from build123d import *

# Parameters (mm, degrees)
F0_W      = 69.0672509372
F0_H      = 104.8798933625
F1_DEPTH  = 25.4
F2_W      = 61.0817540437
F2_H      = 44.6812286973
F3_DEPTH  = 5.08
F5_R      = 6.6887407384
F6_DEPTH  = 25.4
F7_R      = 3.582784906
F8_DEPTH  = 25.4
F9_W      = 4.2634103447
F9_H      = 5.4003186524
F9_W_2    = 5.400320515
F9_H_2    = 4.2634103447
F9_W_3    = 5.1160920411
F9_H_3    = 5.4003195837
F10_DEPTH = 2.286
F4_R      = 4.3385405976
F4_R_2    = 4.6616734777
F11_DEPTH = 2.032
F14_DEPTH = 0.635


with BuildPart() as f1:
    # F0 (on Top) → F1 (new body)
    with BuildSketch(Plane.XY):
        with Locations((-0.2842266113, 5.2582062781)):
            Rectangle(F0_W, F0_H)
    extrude(amount=F1_DEPTH)

    # F2 (on face) → F3 (cut)
    with BuildSketch(Plane.XY.offset(25.4)):
        with Locations((-0.3880532458, 30.3628817201)):
            Rectangle(F2_W, F2_H)
    extrude(amount=-F3_DEPTH, mode=Mode.SUBTRACT)

    # F5 (on Top) → F6 (join)
    with BuildSketch(Plane.XY):
        with Locations((-34.5117151737, 57.5216077268)):
            Circle(F5_R)
    extrude(amount=F6_DEPTH)

    # F7 (on face) → F8 (cut)
    with BuildSketch(Plane.XY.offset(25.4)):
        with Locations((-34.5117151737, 57.5216077268)):
            Circle(F7_R)
    extrude(amount=-F8_DEPTH, mode=Mode.SUBTRACT)

    # F9 (on face) → F10 (join)
    with BuildSketch(Plane.XY.offset(25.4)):
        with Locations((-18.1905506179, -23.1645293534)):
            Rectangle(F9_W, F9_H)
        with Locations((-23.0224160478, -18.3326648548)):
            Rectangle(F9_W_2, F9_H_2)
        with Locations((-18.1905506179, -18.3326648548)):
            Rectangle(F9_W, F9_H_2)
        with Locations((-13.5007994249, -18.3326648548)):
            Rectangle(F9_W_3, F9_H_2)
        with Locations((-18.1905506179, -13.5007998906)):
            Rectangle(F9_W, F9_H_3)
    extrude(amount=F10_DEPTH)

    # F4 (on face) → F11 (join)
    with BuildSketch(Plane.XY.offset(25.4)):
        with Locations((7.2477986105, -11.08486671)):
            Circle(F4_R)
        with Locations((18.3326639235, -4.2634103447)):
            Circle(F4_R_2)
    extrude(amount=F11_DEPTH)

    # F12 (on face) + F13 (on face) → F14 (join)
    with BuildSketch(Plane.XY.offset(25.4)):
        Polygon((5.6323851459, -22.5031040609), (4.3169683777, -21.1328770965), (-1.1299567856, -25.4363407869), (0, -26.8878247589), align=None)
    with BuildSketch(Plane.XY.offset(25.4)):
        Polygon((-10.0978044793, -26.4493525028), (-4.3428572826, -21.790586412), (-5.4735084007, -20.5657135335), (-11.1444314917, -25.1564601203), align=None)
    extrude(amount=F14_DEPTH)


solid = f1.part
The listing builds one solid part. Answer for the finished solid, in the listing's coordinates (mm). A direction names the side the tool comes from. Give positions to 0.01 mm unless a question says otherwise; leave off trailing zeros. Loops run counter-clockwise (first coordinate to the right, second up) from the corner with the lowest first, then second, coordinate; pieces in that order, holes last. Notation, with made-up numbers: (3, -7) - (36, -7) arc R33 ccw to (36, 28) - close; hole circle Ø6 at (-22, 63). An arc over 180 degrees is marked (long way). Use one line per item in the form item = value.
1. Which of the six approach directions +Z, -Z, +X, -X, +Y, -Y give full straight-line access (tool end or side, diameter ignored) to faces 5 (the face through (-18, -10.801, 27)), 6 (the face through (0, 52.703, 23)), 7 (the face through (-39.038, 62.446, 12.522)), 8 (the face through (-13, -16.201, 27)), 9 (the face through (2, -24, 26.035))?
Calculated:
face_5 = +Z, -X, +Y
face_6 = +Z
face_7 = +Z, -Z
face_8 = +Z, +X, +Y
face_9 = +Z, +X, -Y
2. Find the intervals of material crossed by line 1 along Y through (x, z) = (11, 23.75); line 2 along Y through (x, z) = (-4, 11.75); line 3 along Z through (x, y) = (-14, 26), in increasing order. Write a range as [from, to].
Calculated:
line_1 = [-47.18, 8.02], [52.7, 57.7]
line_2 = [-47.18, 57.7]
line_3 = [0, 20.32]
3. Given pin 1 Ø6 at (x, z) = (-16.5, 4) entering from +Y; pin 2 Ø1.8 at (y, z) = (-19.5, 27) entering from -X; pin 3 Ø0.7 at (y, z) = (-13, 27) entering from -X, each flat-ended and moving along its own axis, determine where each tip first touches the part or whether it passes through.
Calculated:
pin_1 = 57.7
pin_2 = -25.72
pin_3 = -20.32
4. Section D-D on y = -39 is taken. Give the vertices of the cut face in (x, z).
Calculated:
outline = (-34.82, 0) - (34.25, 0) - (34.25, 25.4) - (-34.82, 25.4) - close
5. The mould has two halves that part along X. Classify faces 1 (the face through (-10.943, -18, 27)), 2 (the face through (-30.929, 30, 23)), 3 (the face through (-8, -23, 26.035)), 4 (the face through (-1, 31, 20.32)): pulls with the +X half, pulls with the -X half, needs draft (parallel to the pull), parting line crosses it, or undercut.
Calculated:
face_1 = pulls with the +X half
face_2 = undercut
face_3 = needs draft
face_4 = undercut
6. Section C-C on z = 7.5 is taken. Give the vertices of the cut face in (x, y).
Calculated:
outline = (-34.82, -47.18) - (34.25, -47.18) - (34.25, 57.7) - (-27.83, 57.7) arc R6.69 ccw (long way) to (-34.82, 50.84) - close; hole circle Ø7.17 at (-34.51, 57.52)
7. Section B-B on y = 23.5 is taken. Give the vertices of the cut face in (x, z).
Calculated:
outline = (-34.82, 0) - (34.25, 0) - (34.25, 25.4) - (30.15, 25.4) - (30.15, 20.32) - (-30.93, 20.32) - (-30.93, 25.4) - (-34.82, 25.4) - close
8. Section A-A on z = 22.75 is taken. Give the vertices of the cut face in (x, y), then the cut area to 3 significant figures.
Calculated:
outline = (-34.82, -47.18) - (34.25, -47.18) - (34.25, 57.7) - (-27.83, 57.7) arc R6.69 ccw (long way) to (-34.82, 50.84) - close; hole circle Ø7.17 at (-34.51, 57.52); hole (-30.93, 8.02) - (30.15, 8.02) - (30.15, 52.7) - (-29.87, 52.7) arc R6.69 cw to (-30.93, 51.87) - close
area = 4,580 mm^2
